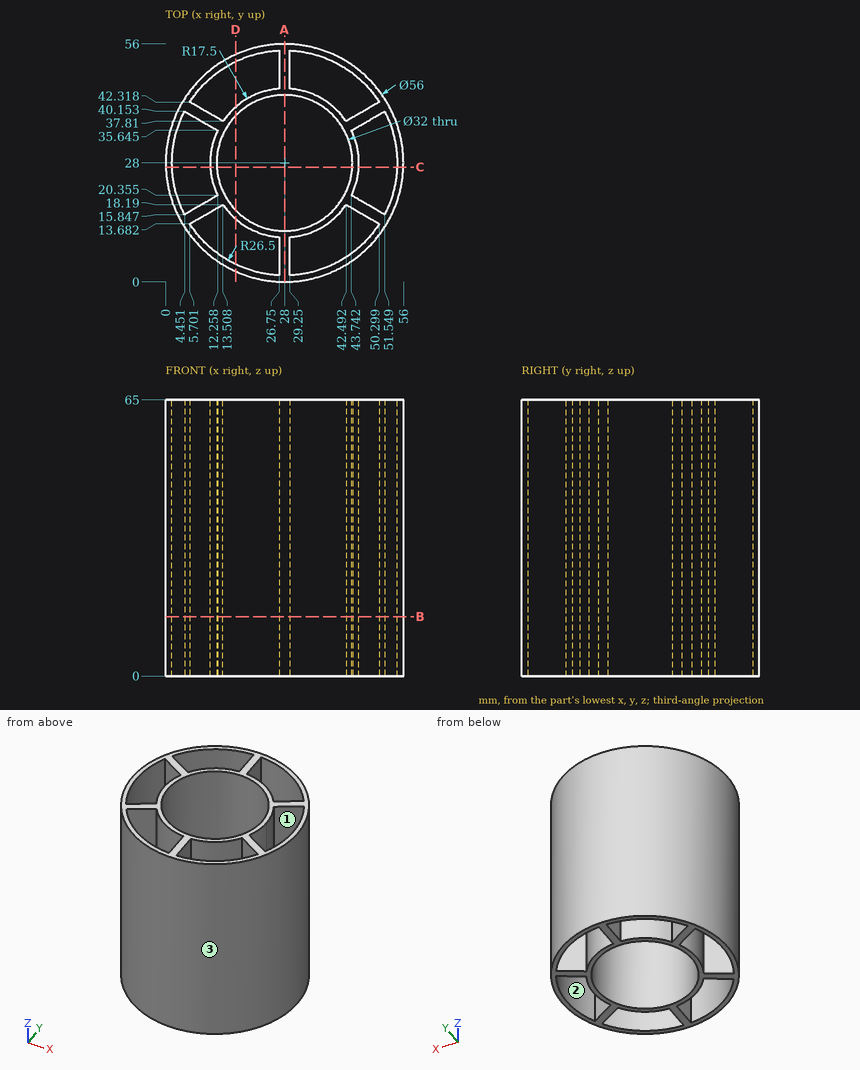
Here's the drawing with two shaded views (mm, measured from the low corner). I have some questions. Round coordinates to 2 decimals unless told otherwise and drop trailing zeros. Write each loop counter-clockwise with the first axis right and the second up, starting at its lowest first coordinate (ties: lowest second). Pieces come first, ordered by that corner, then holes.
(1) Suppose I cut it at A-A on x = 28. Write out the boundary of the cut face in (y, z).
Findings below:
outline: (0, 0) - (12, 0) - (12, 65) - (0, 65) - close; (44, 0) - (56, 0) - (56, 65) - (44, 65) - close
(2) Thinking about a two-plate mould opening in X: for the marked faces 1, 2 and 3, which applies, +X half, -X half, draft (parallel to the pull), parting line (faces both ways), or undercut?
Findings below:
face 1: undercut
face 2: undercut
face 3: parting line
(3) If I drill on probe 1 along Y at (x, z) = (28, 39); probe 2 along Y at (x, z) = (18, 19); probe 3 along X at (y, z) = (20, 54.5) (1 decimal), over which ranges is the centre line in solid material (lowest first)?
Findings below:
probe 1: y = 0 to 12, 44 to 56
probe 2: y = 1.85 to 3.46, 13.64 to 15.51, 40.49 to 42.36, 52.54 to 54.15
probe 3: x = 1.2 to 2.7, 11.6 to 14.1, 41.9 to 44.4, 53.3 to 54.8
(4) Suppose I cut it at C-C on y = 27. Write out the boundary of the cut face in (x, z).
Findings below:
outline: (0.02, 0) - (1.52, 0) - (1.52, 65) - (0.02, 65) - close; (10.53, 0) - (12.03, 0) - (12.03, 65) - (10.53, 65) - close; (43.97, 0) - (45.47, 0) - (45.47, 65) - (43.97, 65) - close; (54.48, 0) - (55.98, 0) - (55.98, 65) - (54.48, 65) - close
(5) Suppose I cut it at B-B on z = 14. State how many separate pieces and enclosed holes the cut face has.
Findings below:
separate pieces: 1
enclosed holes: 7
(6) Suppose I cut it at D-D on x = 16.5. Write out the boundary of the cut face in (y, z) (1 decimal).
Findings below:
outline: (2.5, 0) - (4.1, 0) - (4.1, 65) - (2.5, 65) - close; (14.8, 0) - (16.9, 0) - (16.9, 65) - (14.8, 65) - close; (39.1, 0) - (41.2, 0) - (41.2, 65) - (39.1, 65) - close; (51.9, 0) - (53.5, 0) - (53.5, 65) - (51.9, 65) - close
(7) For pin 1 (1 mm diameter, centred on y = 10.5, z = 49.5, fed in from +X); pin 2 (5 mm diameter, centred on x = 9, z = 6.5, fed in from +Y); pin 3 (7 mm diameter, centred on y = 51.5, z = 45.5, fed in from +X) (1 decimal); pin 4 (1.5 mm diameter, centred on x = 45, y = 10.5, fed in from +Z), each with a flat end and sliding along its axis, tell me the tip position at first contact or that it passes through.
Findings below:
pin 1: stops at x = 50.25
pin 2: stops at y = 50.62
pin 3: stops at x = 47.6
pin 4: passes through
